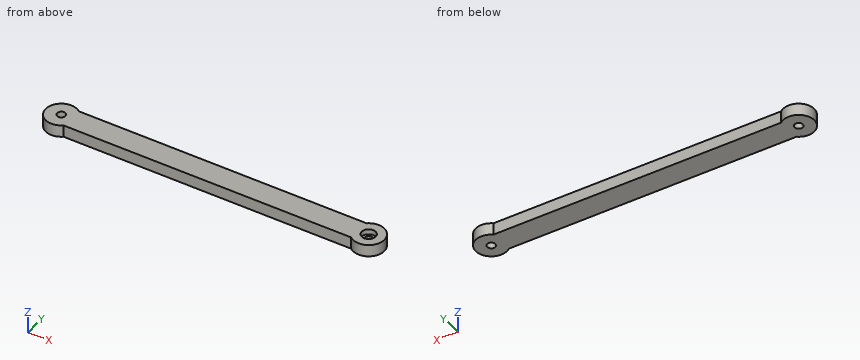
from build123d import *

# Parameters (mm, degrees)
BOSS_EXTRUDE1_START     = -3
SKETCH1_W               = 130
SKETCH1_H               = 10
BOSS_EXTRUDE1_DEPTH     = 5
BOSS_EXTRUDE2_START     = -3
SKETCH2_R               = 6.5
BOSS_EXTRUDE2_DEPTH     = 5
BOSS_EXTRUDE3_START     = -3
SKETCH3_R               = 6.5
BOSS_EXTRUDE3_DEPTH     = 5
CUT_EXTRUDE1_DEPTH      = 137.687600023
CUT_EXTRUDE1_DEPTH_BACK = 137.687600023
SKETCH4_R               = 1.725
CUT_EXTRUDE2_START      = -0.2
SKETCH5_R               = 2.9
CUT_EXTRUDE2_DEPTH      = 2.2


with BuildPart() as part:
    # Sketch1 → Boss-Extrude1 (new body)
    with BuildSketch(Plane.XY.offset(BOSS_EXTRUDE1_START)):
        with Locations((65, 0)):
            Rectangle(SKETCH1_W, SKETCH1_H)
    extrude(amount=BOSS_EXTRUDE1_DEPTH)

    # Sketch2 → Boss-Extrude2 (add)
    with BuildSketch(Plane.XY.offset(BOSS_EXTRUDE2_START)):
        Circle(SKETCH2_R)
    extrude(amount=BOSS_EXTRUDE2_DEPTH)

    # Sketch3 → Boss-Extrude3 (add)
    with BuildSketch(Plane.XY.offset(BOSS_EXTRUDE3_START)):
        with Locations((130, 0)):
            Circle(SKETCH3_R)
    extrude(amount=BOSS_EXTRUDE3_DEPTH)

    # Sketch4 → Cut-Extrude1 (cut, two sides: drawn at the far end of the back side and taken through both)
    with BuildSketch(Plane.XY.offset(-CUT_EXTRUDE1_DEPTH_BACK)):
        Circle(SKETCH4_R)
        with Locations((130, 0)):
            Circle(SKETCH4_R)
    extrude(amount=CUT_EXTRUDE1_DEPTH + CUT_EXTRUDE1_DEPTH_BACK, mode=Mode.SUBTRACT)

    # Sketch5 → Cut-Extrude2 (cut)
    with BuildSketch(Plane.XY.offset(CUT_EXTRUDE2_START)):
        with Locations((130, 0)):
            Circle(SKETCH5_R)
    extrude(amount=CUT_EXTRUDE2_DEPTH, mode=Mode.SUBTRACT)


solid = part.part
CAD build for the part. Positions are in the model's coordinates, mm. Round coordinates to 2 decimals unless told otherwise and drop trailing zeros. Write each loop counter-clockwise with the first axis right and the second up, starting at its lowest first coordinate (ties: lowest second). Pieces come first, ordered by that corner, then holes. Notation, with made-up numbers: M 50.25,33.5 L 61.25,33.5 A23 ccw 61.25,60.5 Z; hole C 24,19.5 d4. An arc over 180 degrees is marked long. Put each result on its own line as item: value. Start each with the question number.
1) Saw through at A-A, the plane x = 0. Write the cut outline in (y, z) (3 decimals), and give its area (4 significant figures).
2) Pin check, flat tips, straight feed: pin 1 Ø3 at (y, z) = (3.5, 1.5) entering from +X; pin 2 Ø1.5 at (x, z) = (63, -1) entering from -Y. Stop position of each tip, or through.
3) Drill centre lines: probe 1 along X at (y, z) = (0, -0.7) (3 decimals); probe 2 along Y at (x, z) = (0, 0.3) (3 decimals); probe 3 along X at (y, z) = (-1.5, -1.55). Where is each one in solid material? Low to high. Write a range as [from, to].
4) Saw through at D-D, the plane x = 130. Write the cut outline in (y, z) (3 decimals), and give its area (3 significant figures).
5) Saw through at C-C, the plane z = 1. Write the cut outline in (x, y) (3 decimals), and give its area (3 significant figures).
6) Saw through at B-B, the plane y = 0. Write the cut outline in (x, z) (3 decimals).
Resolved:
1. outline: M -6.5,-3 L -1.725,-3 L -1.725,2 L -6.5,2 Z; M 1.725,-3 L 6.5,-3 L 6.5,2 L 1.725,2 Z
1. area: 47.75 mm²
2. pin 1: x = 136.18
2. pin 2: y = -5
3. probe 1: [-6.5, -1.725], [1.725, 128.275], [131.725, 136.5]
3. probe 2: [-6.5, -1.725], [1.725, 6.5]
3. probe 3: [-6.32, -0.85], [0.85, 129.15], [130.85, 136.32]
4. outline: M -6.5,-3 L -1.725,-3 L -1.725,-0.2 L -2.9,-0.2 L -2.9,2 L -6.5,2 Z; M 1.725,-3 L 6.5,-3 L 6.5,2 L 2.9,2 L 2.9,-0.2 L 1.725,-0.2 Z
4. area: 42.6 mm²
5. outline: M 4.153,-5 L 125.847,-5 A6.5 ccw long 125.847,5 L 4.153,5 A6.5 ccw long Z; hole C 0,0 d3.45; hole C 130,0 d5.8
5. area: 1,410 mm²
6. outline: M -6.5,-3 L -1.725,-3 L -1.725,2 L -6.5,2 Z; M 1.725,-3 L 128.275,-3 L 128.275,-0.2 L 127.1,-0.2 L 127.1,2 L 1.725,2 Z; M 131.725,-3 L 136.5,-3 L 136.5,2 L 132.9,2 L 132.9,-0.2 L 131.725,-0.2 Z
